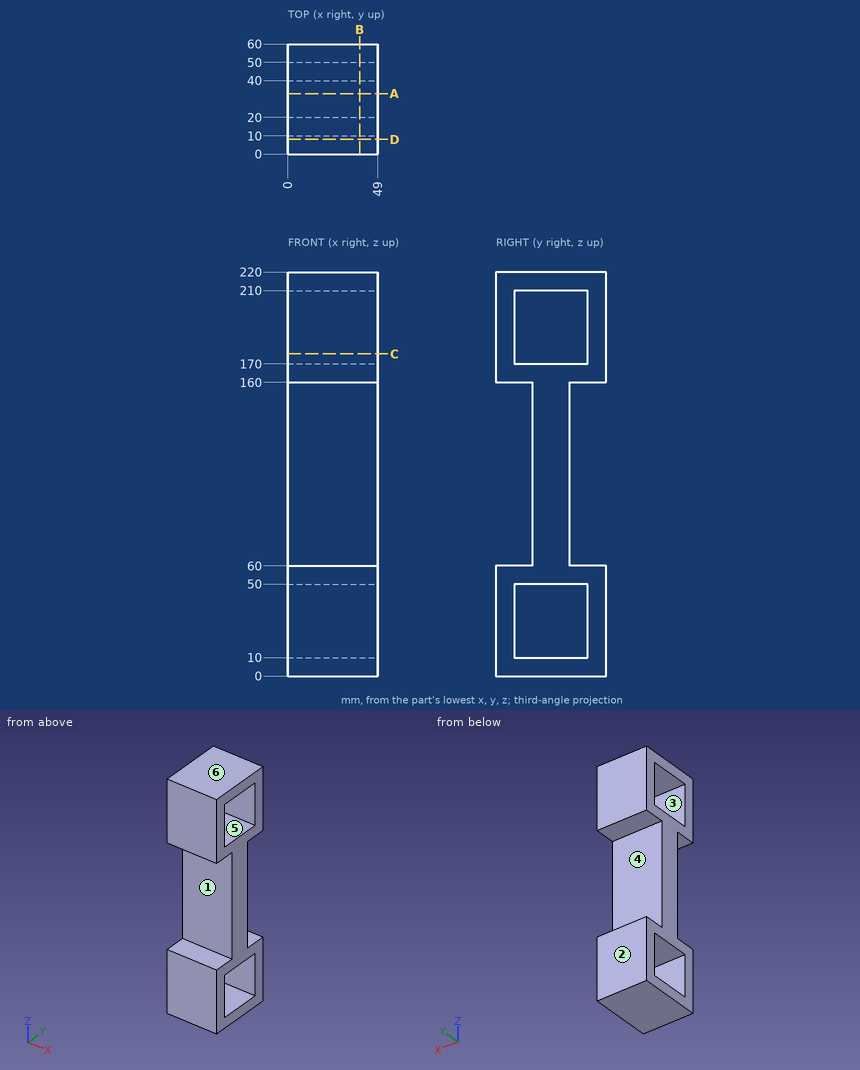
The drawing under review shows one solid part. Ordinate dimensions are in mm from its lowest x, y, z. A direction names the side the tool comes from. Give positions to 0.01 mm unless a question says otherwise; leave off trailing zeros. Write each loop counter-clockwise with the first axis right and the second up, starting at its lowest first coordinate (ties: lowest second). Pieces come first, ordered by that corner, then holes. Notation, with made-up numbers: (-19.5, -29) - (-5.5, -29) arc R20 cw to (-5.5, -24) - close; hole circle Ø5 at (-35, 63.5). An arc over 180 degrees is marked (long way). Answer in a Markdown table with one row per item. Add a question column.
1. We need section D-D on y = 8. Write out the cut boundary in (x, z).
2. We need section C-C on z = 175.5. Write out the cut boundary in (x, y), then the cut area to 3 significant figures.
3. Wall thickness on line 1 along Z through (x, y) = (36, 27.5); line 2 along Z through (x, y) = (28.5, 46); line 3 along Z through (x, y) = (18, 6): over which ranges is each line inside the solid? List them lowest first. Write a range as [from, to].
4. Insertion check: P1, Ø14.5, axis at x = 18, z = 104, coming from the -Y side. The pin has a flat end and moves straight along its axis. Give the tip position at first contact, or say it passes through.
5. We need section A-A on y = 33. Write out the cut boundary in (x, z), then the cut area to 3 significant figures.
6. Draft analysis for pull direction Y (two halves, no side actions). For the marked faces 1, 2 and 3, state which applies: +Y half, -Y half, draft (parallel to the pull), parting line (faces both ways), or undercut.
7. We need section B-B on x = 39. Write out the cut boundary in (y, z), then the cut area to 3 significant figures.
8. Tool access review of the marked faces 4, 5 and 6: name each direction out of +Z, -Z, +X, -X, +Y, -Y from which nothing blocks a thin tool from reaching the whole face with its end or side.
Ans:
| question | item | result |
|---|---|---|
| 1 | outline | (0, 0) - (49, 0) - (49, 60) - (0, 60) - close; (0, 160) - (49, 160) - (49, 220) - (0, 220) - close |
| 2 | outline | (0, 0) - (49, 0) - (49, 10) - (0, 10) - close; (0, 50) - (49, 50) - (49, 60) - (0, 60) - close |
| 2 | area | 980 mm^2 |
| 3 | line 1 | z = [0, 10], [50, 170], [210, 220] |
| 3 | line 2 | z = [0, 10], [50, 60], [160, 170], [210, 220] |
| 3 | line 3 | z = [0, 60], [160, 220] |
| 4 | P1 | stops at y = 20 |
| 5 | outline | (0, 0) - (49, 0) - (49, 10) - (0, 10) - close; (0, 50) - (49, 50) - (49, 170) - (0, 170) - close; (0, 210) - (49, 210) - (49, 220) - (0, 220) - close |
| 5 | area | 6,860 mm^2 |
| 6 | face 1 | -Y half |
| 6 | face 2 | +Y half |
| 6 | face 3 | undercut |
| 7 | outline | (0, 0) - (60, 0) - (60, 60) - (40, 60) - (40, 160) - (60, 160) - (60, 220) - (0, 220) - (0, 160) - (20, 160) - (20, 60) - (0, 60) - close; hole (10, 10) - (50, 10) - (50, 50) - (10, 50) - close; hole (10, 170) - (50, 170) - (50, 210) - (10, 210) - close |
| 7 | area | 6,000 mm^2 |
| 8 | face 4 | +X, -X, +Y |
| 8 | face 5 | +X, -X |
| 8 | face 6 | +Z, +X, -X, +Y, -Y |
